from build123d import *

# Parameters (mm, degrees)
SKETCH1_W           = 70.9
SKETCH1_H           = 143.6
BOSS_EXTRUDE1_DEPTH = 7.7
FILLET1_R           = 9
BOSS_EXTRUDE2_DEPTH = 1.7
BOSS_EXTRUDE3_DEPTH = 1.7
SKETCH4_W           = 3.333340828
SKETCH4_H           = 6.136400457
CUT_EXTRUDE1_DEPTH  = 1.7
SKETCH5_W           = 1.382906497
SKETCH5_H           = 5.927261181
BOSS_EXTRUDE4_DEPTH = 1.7
BOSS_EXTRUDE5_DEPTH = 1.7
SKETCH7_R           = 1.766648845
CUT_EXTRUDE2_DEPTH  = 0.7
CUT_EXTRUDE3_DEPTH  = 6.7
SKETCH9_R           = 1.234780667
CUT_EXTRUDE4_DEPTH  = 4.7
LPATTERN1_COUNT     = 5
LPATTERN1_PITCH     = 4
SKETCH10_R          = 1.403334483
CUT_EXTRUDE5_DEPTH  = 4.7
LPATTERN2_COUNT     = 5
LPATTERN2_PITCH     = 4
CUT_EXTRUDE6_DEPTH  = 2.7
FILLET2_R           = 1.7
FILLET3_R           = 1.7


with BuildPart() as part:
    # Sketch1 → Boss-Extrude1 (new body)
    with BuildSketch(Plane.XY):
        with Locations((35.45, -71.8)):
            Rectangle(SKETCH1_W, SKETCH1_H)
    extrude(amount=BOSS_EXTRUDE1_DEPTH)

    # Fillet1
    fillet1_edges = [part.edges().sort_by_distance(p)[0] for p in [
        (0, 0, 3.85),
        (70.9, 0, 3.85),
        (70.9, -143.6, 3.85),
        (0, -143.6, 3.85),
    ]]
    fillet(fillet1_edges, radius=FILLET1_R)

    # Sketch2 → Boss-Extrude2 (add)
    with BuildSketch(Plane(origin=(70.9, -8.327936867, 0), x_dir=(0, 0, -1), z_dir=(1, 0, 0))):
        with BuildLine():
            Line((-5.605090694, -45.631969305), (-5.605090694, -25.092533891))
            ThreePointArc((-5.605090694, -25.092533891), (-3.85, -23.337443197), (-2.094909306, -25.092533891))
            Line((-2.094909306, -25.092533891), (-2.094909306, -45.631969305))
            ThreePointArc((-2.094909306, -45.631969305), (-3.85, -47.387059999), (-5.605090694, -45.631969305))
        make_face()
    extrude(amount=BOSS_EXTRUDE2_DEPTH)

    # Sketch3 → Boss-Extrude3 (add)
    with BuildSketch(Plane.ZY):
        with BuildLine():
            ThreePointArc((5.711355616, -60.986538732), (3.85, -62.847894348), (1.988644384, -60.986538732))
            Line((1.988644384, -60.986538732), (1.988644384, -49.990125604))
            ThreePointArc((1.988644384, -49.990125604), (3.85, -48.128769988), (5.711355616, -49.990125604))
            Line((5.711355616, -49.990125604), (5.711355616, -60.986538732))
        make_face()
        with BuildLine():
            ThreePointArc((5.711355616, -31.75341953), (3.85, -29.892063915), (1.988644384, -31.75341953))
            Line((1.988644384, -31.75341953), (1.988644384, -42.749832659))
            ThreePointArc((1.988644384, -42.749832659), (3.85, -44.611188275), (5.711355616, -42.749832659))
            Line((5.711355616, -42.749832659), (5.711355616, -31.75341953))
        make_face()
    extrude(amount=BOSS_EXTRUDE3_DEPTH)

    # Sketch4 → Cut-Extrude1 (cut)
    with BuildSketch(Plane.ZY):
        with Locations((3.85, -22.514232186)):
            Rectangle(SKETCH4_W, SKETCH4_H)
    extrude(amount=-CUT_EXTRUDE1_DEPTH, mode=Mode.SUBTRACT)

    # Sketch5 → Boss-Extrude4 (add)
    with BuildSketch(Plane.ZY.offset(-1.7)):
        with Locations((3.095312634, -22.618801824)):
            Rectangle(SKETCH5_W, SKETCH5_H)
    extrude(amount=BOSS_EXTRUDE4_DEPTH)

    # Sketch6 → Boss-Extrude5 (add)
    with BuildSketch(Plane(origin=(0, 0, 0), x_dir=(-1, 0, 0), z_dir=(0, 0, -1))):
        with BuildLine():
            ThreePointArc((-58.291417144, -28.459192447), (-62.200913295, -32.368688598), (-66.110409446, -28.459192447))
            Line((-66.110409446, -28.459192447), (-66.110409446, -9.312433578))
            ThreePointArc((-66.110409446, -9.312433578), (-62.200913295, -5.402937427), (-58.291417144, -9.312433578))
            Line((-58.291417144, -9.312433578), (-58.291417144, -28.459192447))
        make_face()
    extrude(amount=BOSS_EXTRUDE5_DEPTH)

    # Sketch7 → Cut-Extrude2 (cut)
    with BuildSketch(Plane(origin=(0, 0, -1.7), x_dir=(-1, 0, 0), z_dir=(0, 0, -1))):
        with Locations((-62.200913295, -18.885813012)):
            Circle(SKETCH7_R)
    extrude(amount=-CUT_EXTRUDE2_DEPTH, mode=Mode.SUBTRACT)

    # Sketch8 → Cut-Extrude3 (cut)
    with BuildSketch(Plane(origin=(0, -143.6, 0), x_dir=(-1, 0, 0), z_dir=(0, -1, 0))):
        with BuildLine():
            Line((-32.382593944, -2.596190666), (-38.517406056, -2.596190666))
            ThreePointArc((-38.517406056, -2.596190666), (-39.77121539, -3.85), (-38.517406056, -5.103809334))
            Line((-38.517406056, -5.103809334), (-32.382593944, -5.103809334))
            ThreePointArc((-32.382593944, -5.103809334), (-31.12878461, -3.85), (-32.382593944, -2.596190666))
        make_face()
    extrude(amount=-CUT_EXTRUDE3_DEPTH, mode=Mode.SUBTRACT)

    # Sketch9 → Cut-Extrude4 (cut)
    with BuildSketch(Plane.XZ.offset(143.6)):
        with Locations(Location((44.624064911, 3.85, 0), (0, 0, 270))):
            Circle(SKETCH9_R)
    cut_extrude4 = extrude(amount=-CUT_EXTRUDE4_DEPTH, mode=Mode.SUBTRACT)

    # LPattern1: Cut-Extrude4 ×5
    with Locations(*[(i * LPATTERN1_PITCH, 0, 0) for i in range(1, LPATTERN1_COUNT)]):
        add(cut_extrude4, mode=Mode.SUBTRACT)

    # Sketch10 → Cut-Extrude5 (cut)
    with BuildSketch(Plane.XZ.offset(143.6)):
        with Locations(Location((26.034503903, 3.85, 0), (0, 0, 270))):
            Circle(SKETCH10_R)
    cut_extrude5 = extrude(amount=-CUT_EXTRUDE5_DEPTH, mode=Mode.SUBTRACT)

    # LPattern2: Cut-Extrude5 ×5
    with Locations(*[(-i * LPATTERN2_PITCH, 0, 0) for i in range(1, LPATTERN2_COUNT)]):
        add(cut_extrude5, mode=Mode.SUBTRACT)

    # Sketch11 → Cut-Extrude6 (cut)
    with BuildSketch(Plane(origin=(0, -1.738509759, 7.7), x_dir=(1, 0, 0), z_dir=(0, 0, 1))):
        with BuildLine():
            Line((27.492370642, -3.734093894), (43.158394407, -3.734093894))
            ThreePointArc((43.158394407, -3.734093894), (44.126748247, -2.765740054), (43.158394407, -1.797386213))
            Line((43.158394407, -1.797386213), (27.492370642, -1.797386213))
            ThreePointArc((27.492370642, -1.797386213), (26.524016802, -2.765740054), (27.492370642, -3.734093894))
        make_face()
    extrude(amount=-CUT_EXTRUDE6_DEPTH, mode=Mode.SUBTRACT)

    # Fillet2
    fillet2_edges = [part.edges().sort_by_distance(p)[0] for p in [
        (68.263961031, -2.636038969, 7.7),
        (70.9, -71.8, 7.7),
        (68.263961031, -140.963961031, 7.7),
        (35.45, -143.6, 7.7),
        (2.636038969, -140.963961031, 7.7),
        (0, -71.8, 7.7),
        (2.636038969, -2.636038969, 7.7),
        (35.45, 0, 7.7),
    ]]
    fillet(fillet2_edges, radius=FILLET2_R)

    # Fillet3
    fillet3_edges = [part.edges().sort_by_distance(p)[0] for p in [
        (35.45, -143.6, 0),
        (0, -71.8, 0),
        (35.45, 0, 0),
        (70.9, -71.8, 0),
        (68.263961031, -2.636038969, 0),
        (2.636038969, -2.636038969, 0),
        (68.263961031, -140.963961031, 0),
        (2.636038969, -140.963961031, 0),
    ]]
    fillet(fillet3_edges, radius=FILLET3_R)


solid = part.part
The listing builds one solid part. Answer for the finished solid, in the listing's coordinates (mm). A direction names the side the tool comes from. Give positions to 0.01 mm unless a question says otherwise; leave off trailing zeros. Write each loop counter-clockwise with the first axis right and the second up, starting at its lowest first coordinate (ties: lowest second). Pieces come first, ordered by that corner, then holes. Notation, with made-up numbers: (-36, 22.25) -> (22, 22.25) arc R11 cw to (22, 39.25) -> close; hole circle Ø8 at (53, -22.5). An arc over 180 degrees is marked (long way). Use a Markdown table: item, result.
(1) For faces 5 (the flat face through (62, -19, -1)), 6 (the cylindrical face through (49.85, -141.28, 4.01)), 7 (the flat face through (35, -5.473, 6)), determine the directions among +Z, -Z, +X, -X, +Y, -Y from which every point of the face is accessible in a straight line to the end or side of a thin tool.
Return value:
| item | result |
|---|---|
| face 5 | -Z |
| face 6 | -Y |
| face 7 | +Z |
(2) Find the intervals of material crossed by probe 1 along X at (y, z) = (-90, 1.5); probe 2 along Y at (x, z) = (26, 3.75); probe 3 along Z at (x, y) = (62, -71.5), in increasing order. Write a range as from..to.
Return value:
| item | result |
|---|---|
| probe 1 | 0.01..70.89 |
| probe 2 | -138.9..0 |
| probe 3 | 0..7.7 |
(3) Flat-ended cylindrical pins translate along their axes: P1, Ø0.8, axis at x = 17.5, z = 4.5, coming from the -Y side; P2, Ø1.5, axis at x = 34, y = -4.5, coming from the +Z side; P3, Ø1.4, axis at x = 1, y = -23.5, coming from the -Z side. Find the tip coordinate at first contact, or state that the pin passes through.
Return value:
| item | result |
|---|---|
| P1 | y = -138.9 |
| P2 | z = 5 |
| P3 | z = 0 |
(4) Determine the mould class of faces 1 (the flat face through (22, -138.9, 4)), 2 (the flat face through (35, -3.536, 6)), 3 (the flat face through (35, -140, 2.596)), 4 (the cylindrical face through (63.966, -18.808, -1.355)) for opening direction Y: released by +Y, released by -Y, zero draft, split by the parting line, or undercut.
Return value:
| item | result |
|---|---|
| face 1 | released by -Y |
| face 2 | undercut |
| face 3 | zero draft |
| face 4 | undercut |
(5) Section A-A, the plane y = -124 is taken. Determine the outline of the cut face in (x, z).
Return value:
| item | result |
|---|---|
| outline | (0, 1.7) arc R1.7 ccw to (1.7, 0) -> (69.2, 0) arc R1.7 ccw to (70.9, 1.7) -> (70.9, 6) arc R1.7 ccw to (69.2, 7.7) -> (1.7, 7.7) arc R1.7 ccw to (0, 6) -> close |
